Geometry: final body of the model. Coordinates: model frame, mm. Coordinates: 2 decimals unless noted, no trailing zeros. Order: outer loops, then holes, each group sorted by start corner. A loop starts at its lowest first (then second) coordinate and runs counter-clockwise, first axis right, second up. Notation, with made-up numbers: (84.5, 31.5) -> (134.5, 31.5) arc R22 cw to (134.5, 64.5) -> close; hole circle Ø10 at (-21.75, 33). An arc over 180 degrees is marked (long way). Use one line per item in the form item = value.
```python
from build123d import *

# Parameters (mm, degrees)
F1_DEPTH = 5.08


with BuildPart() as f1:
    # F0 (on Front) → F1 (new body)
    with BuildSketch(Plane.XZ):
        with BuildLine():
            Line((53.975, 0), (0, 0))
            Line((0, 0), (-53.975, 0))
            ThreePointArc((-53.975, 0), (-56.7648079092, -6.7351920908), (-63.5, -9.525))
            Line((-63.5, -9.525), (63.5, -9.525))
            ThreePointArc((63.5, -9.525), (56.7648079092, -6.7351920908), (53.975, 0))
        make_face()
        with BuildLine():
            Line((-53.975, 0), (0, 0))
            Line((0, 0), (53.975, 0))
            ThreePointArc((53.975, 0), (56.7648079092, 6.7351920908), (63.5, 9.525))
            Line((63.5, 9.525), (-63.5, 9.525))
            ThreePointArc((-63.5, 9.525), (-56.7648079092, 6.7351920908), (-53.975, 0))
        make_face()
        with BuildLine():
            ThreePointArc((-63.5, -9.525), (-56.7648079092, -6.7351920908), (-53.975, 0))
            Line((-53.975, 0), (-57.15, 0))
            ThreePointArc((-57.15, 0), (-59.0098719395, -4.4901280605), (-63.5, -6.35))
            Line((-63.5, -6.35), (-63.5, -9.525))
        make_face()
        with BuildLine():
            Line((-57.15, 0), (-53.975, 0))
            ThreePointArc((-53.975, 0), (-56.7648079092, 6.7351920908), (-63.5, 9.525))
            Line((-63.5, 9.525), (-63.5, 6.35))
            ThreePointArc((-63.5, 6.35), (-59.0098719395, 4.4901280605), (-57.15, 0))
        make_face()
        with BuildLine():
            ThreePointArc((63.5, 9.525), (56.7648079092, 6.7351920908), (53.975, 0))
            Line((53.975, 0), (57.15, 0))
            ThreePointArc((57.15, 0), (59.0098719395, 4.4901280605), (63.5, 6.35))
            Line((63.5, 6.35), (63.5, 9.525))
        make_face()
        with BuildLine():
            Line((57.15, 0), (53.975, 0))
            ThreePointArc((53.975, 0), (56.7648079092, -6.7351920908), (63.5, -9.525))
            Line((63.5, -9.525), (63.5, -6.35))
            ThreePointArc((63.5, -6.35), (59.0098719395, -4.4901280605), (57.15, 0))
        make_face()
        with BuildLine():
            Line((-63.5, 6.35), (-63.5, 9.525))
            ThreePointArc((-63.5, 9.525), (-73.025, 0), (-63.5, -9.525))
            Line((-63.5, -9.525), (-63.5, -6.35))
            ThreePointArc((-63.5, -6.35), (-69.85, 0), (-63.5, 6.35))
        make_face()
        with BuildLine():
            ThreePointArc((73.025, 0), (70.2351920908, 6.7351920908), (63.5, 9.525))
            Line((63.5, 9.525), (63.5, 6.35))
            ThreePointArc((63.5, 6.35), (67.9901280605, 4.4901280605), (69.85, 0))
            ThreePointArc((69.85, 0), (67.9901280605, -4.4901280605), (63.5, -6.35))
            Line((63.5, -6.35), (63.5, -9.525))
            ThreePointArc((63.5, -9.525), (70.2351920908, -6.7351920908), (73.025, 0))
        make_face()
    extrude(amount=F1_DEPTH)


solid = f1.part
```
1) Section D-D, the plane z = 8. Output: boundary loops of the cut face in (x, y).
Results found:
outline = (-68.67, -5.08) -> (68.67, -5.08) -> (68.67, 0) -> (-68.67, 0) -> close
2) Contact query for flat-ended pins moving along their axis: P1, Ø1, axis at y = -1, z = 2.5, coming from the +X side; P2, Ø1.5, axis at x = -7.5, z = -4.5, coming from the +Y side. Output: stop coordinate, or through.
Results found:
P1 = 72.81
P2 = 0
3) Section C-C, the plane x = 60. Output: boundary loops of the cut face in (y, z) (3 decimals).
Results found:
outline = (-5.08, -9.525) -> (0, -9.525) -> (0, -5.298) -> (-5.08, -5.298) -> close; (-5.08, 5.298) -> (0, 5.298) -> (0, 9.525) -> (-5.08, 9.525) -> close
4) Section A-A, the plane y = -2.25. Output: boundary loops of the cut face in (x, z) (3 decimals).
Results found:
outline = (-63.5, -9.525) -> (63.5, -9.525) arc R9.525 ccw to (63.5, 9.525) -> (-63.5, 9.525) arc R9.525 ccw to start; hole circle Ø12.7 at (-63.5, 0); hole circle Ø12.7 at (63.5, 0)
5) Material intervals for probe 1 along X at (y, z) = (-3.25, 0.25); probe 2 along X at (y, z) = (-3.65, 4); probe 3 along X at (y, z) = (-4.5, 7.5), sorted ascending. Write a range as from..to.
Results found:
probe_1 = -73.02..-69.85, -57.15..57.15, 69.85..73.02
probe_2 = -72.14..-68.43, -58.57..58.57, 68.43..72.14
probe_3 = -69.37..69.37
6) Section B-B, the plane z = 1.5. Output: boundary loops of the cut face in (x, y).
Results found:
outline = (-72.91, -5.08) -> (-69.67, -5.08) -> (-69.67, 0) -> (-72.91, 0) -> close; (-57.33, -5.08) -> (57.33, -5.08) -> (57.33, 0) -> (-57.33, 0) -> close; (69.67, -5.08) -> (72.91, -5.08) -> (72.91, 0) -> (69.67, 0) -> close
